Could you check a few things on this drawing? It's one solid part, dimensions in mm from its lowest x, y, z. Round coordinates to 2 decimals unless told otherwise and drop trailing zeros. Order: outer loops, then holes, each group sorted by start corner. A loop starts at its lowest first (then second) coordinate and runs counter-clockwise, first axis right, second up. Notation, with made-up numbers: (-12, 63) - (4, 63) arc R26 cw to (4, 101) - close; hole circle Ø8 at (-12.75, 89). An arc over 180 degrees is marked (long way). Use one line per item in the form item = value.
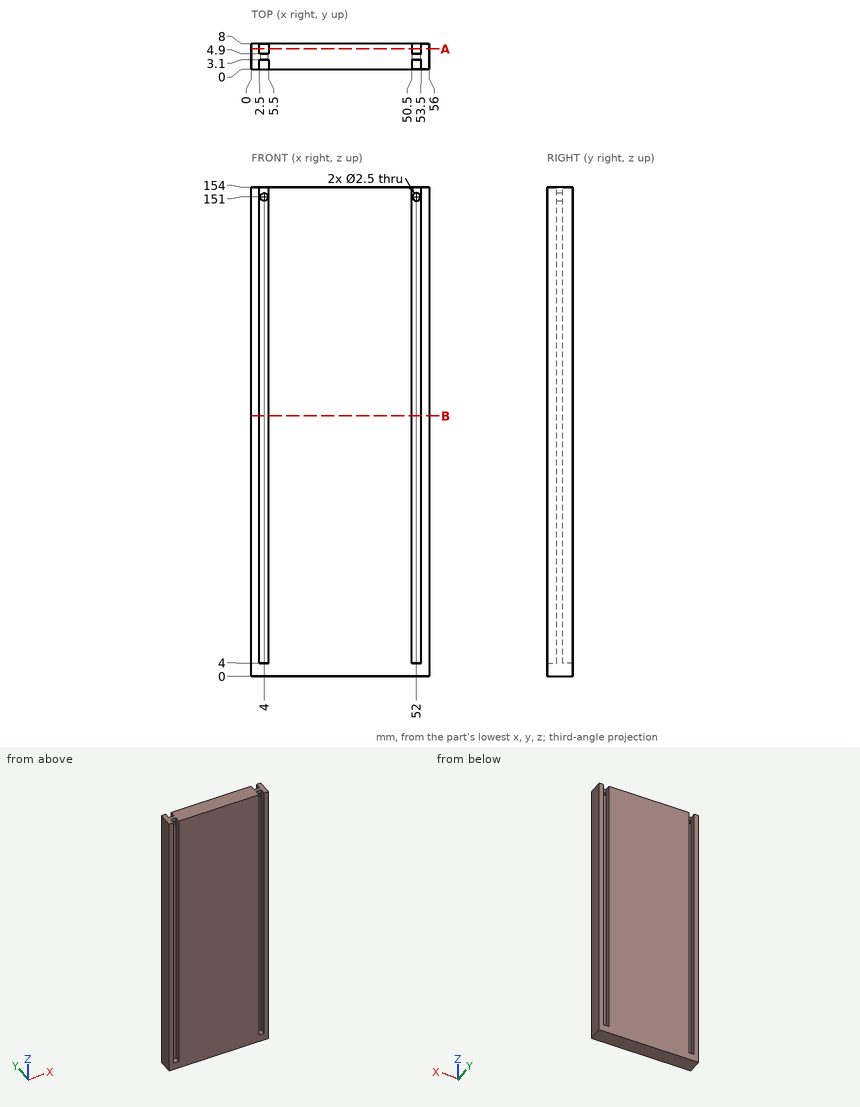
Item 1: Imagine slicing it at B-B on z = 82. Please give me the cut outline in (x, y).
Found:
outline = (0, 0) - (2.5, 0) - (2.5, 3.1) - (5.5, 3.1) - (5.5, 0) - (50.5, 0) - (50.5, 3.1) - (53.5, 3.1) - (53.5, 0) - (56, 0) - (56, 8) - (53.5, 8) - (53.5, 4.9) - (50.5, 4.9) - (50.5, 8) - (5.5, 8) - (5.5, 4.9) - (2.5, 4.9) - (2.5, 8) - (0, 8) - close
Item 2: Will these pins go through, and if not, where does the flat tip stop? P1, Ø3.5, axis at y = 7, z = 83.5, coming from the -X side; P2, Ø1.5, axis at x = 4, y = 1, coming from the +Z side; P3, Ø2.5, axis at x = 4, z = 47, coming from the +Y side.
Found:
P1 = 0
P2 = 4
P3 = 4.9
Item 3: Imagine slicing it at A-A on y = 6.5. Please give me the cut outline in (x, z).
Found:
outline = (0, 0) - (56, 0) - (56, 154) - (53.5, 154) - (53.5, 4) - (50.5, 4) - (50.5, 154) - (5.5, 154) - (5.5, 4) - (2.5, 4) - (2.5, 154) - (0, 154) - close
Item 4: I need wall thicknesses on L1, parallel to X at y = 5.25, z = 30.5; L2, parallel to X at y = 4.55, z = 151; L3, parallel to Z at x = 4, y = 4.2. Which ranges of each line are inside material? Lowest first, please.
Found:
L1 = 0 to 2.5, 5.5 to 50.5, 53.5 to 56
L2 = 0 to 2.75, 5.25 to 50.75, 53.25 to 56
L3 = 0 to 149.75, 152.25 to 154
